Design review of the part built by this model. Coordinates are the model's own, in mm. A direction names the side the tool comes from. Give positions to 0.01 mm unless a question says otherwise; leave off trailing zeros. Loops run counter-clockwise (first coordinate to the right, second up) from the corner with the lowest first, then second, coordinate; pieces in that order, holes last.
from build123d import *

# Parameters (mm, degrees)
F1_DEPTH = 0.508
F3_DEPTH = 2.54
F5_DEPTH = 0.254


with BuildPart() as f1:
    # F0 (on Top) → F1 (new body)
    with BuildSketch(Plane.XY):
        with BuildLine():
            Line((0.5969, 12.4386211307), (0.5969, 13.7155528236))
            ThreePointArc((0.5969, 13.7155528236), (0, 20.3739569369), (-0.5969, 13.7155528236))
            Line((-0.5969, 13.7155528236), (-0.5969, 12.4386211307))
            Line((-0.5969, 12.4386211307), (-6.4008217303, 11.9018768547))
            ThreePointArc((-6.4008217303, 11.9018768547), (-6.1880330513, 11.6046108469), (-6.1128665152, 11.2468454306))
            ThreePointArc((-6.1128665152, 11.2468454306), (-6.1585456161, 10.965543349), (-6.2908886999, 10.7131493128))
            Line((-6.2908886999, 10.7131493128), (-0.5969, 11.2397270277))
            Line((-0.5969, 11.2397270277), (-0.5969, 7.3000811972))
            Line((-0.5969, 7.3000811972), (-3.5388981923, 0))
            Line((-3.5388981923, 0), (-2.2769883957, 0))
            Line((-2.2769883957, 0), (0, 5.6499695401))
            Line((0, 5.6499695401), (2.2769883957, 0))
            Line((2.2769883957, 0), (3.5388981923, 0))
            Line((3.5388981923, 0), (0.5969, 7.3000811972))
            Line((0.5969, 7.3000811972), (0.5969, 11.2397270277))
            Line((0.5969, 11.2397270277), (6.2908886999, 10.7131493128))
            ThreePointArc((6.2908886999, 10.7131493128), (6.1166438776, 11.3287104532), (6.4008217303, 11.9018768547))
            Line((6.4008217303, 11.9018768547), (0.5969, 12.4386211307))
        make_face()
        with BuildLine():
            ThreePointArc((7.8908665152, 11.2468454306), (7.3596319315, 12.0606788944), (6.4008217303, 11.9018768547))
            Line((6.4008217303, 11.9018768547), (7.0568330304, 11.8412092015))
            Line((7.0568330304, 11.8412092015), (6.9469, 10.6524816596))
            Line((6.9469, 10.6524816596), (6.2908886999, 10.7131493128))
            ThreePointArc((6.2908886999, 10.7131493128), (7.2831685968, 10.4035245315), (7.8908665152, 11.2468454306))
        make_face()
        with BuildLine():
            Line((7.0568330304, 11.8412092015), (6.4008217303, 11.9018768547))
            ThreePointArc((6.4008217303, 11.9018768547), (6.1166438776, 11.3287104532), (6.2908886999, 10.7131493128))
            Line((6.2908886999, 10.7131493128), (6.9469, 10.6524816596))
            Line((6.9469, 10.6524816596), (7.0568330304, 11.8412092015))
        make_face()
        with BuildLine():
            ThreePointArc((-6.1128665152, 11.2468454306), (-6.1880330513, 11.6046108469), (-6.4008217303, 11.9018768547))
            Line((-6.4008217303, 11.9018768547), (-7.0568330304, 11.8412092015))
            Line((-7.0568330304, 11.8412092015), (-6.9469, 10.6524816596))
            Line((-6.9469, 10.6524816596), (-6.2908886999, 10.7131493128))
            ThreePointArc((-6.2908886999, 10.7131493128), (-6.1585456161, 10.965543349), (-6.1128665152, 11.2468454306))
        make_face()
        with BuildLine():
            Line((-7.0568330304, 11.8412092015), (-6.4008217303, 11.9018768547))
            ThreePointArc((-6.4008217303, 11.9018768547), (-7.8870891528, 11.164980408), (-6.2908886999, 10.7131493128))
            Line((-6.2908886999, 10.7131493128), (-6.9469, 10.6524816596))
            Line((-6.9469, 10.6524816596), (-7.0568330304, 11.8412092015))
        make_face()
    extrude(amount=F1_DEPTH)

    # F2 (on face) → F3 (join)
    with BuildSketch(Plane.XY.offset(0.508)):
        with BuildLine():
            Line((-3.5388981923, 0), (-2.2769883957, 0))
            ThreePointArc((-2.2769883957, 0), (-2.907943294, 0.6309548983), (-3.5388981923, 0))
        make_face()
        with BuildLine():
            ThreePointArc((3.5388981923, 0), (2.907943294, 0.6309548983), (2.2769883957, 0))
            Line((2.2769883957, 0), (3.5388981923, 0))
        make_face()
    extrude(amount=F3_DEPTH)

    # F4 (on face) → F5 (join)
    with BuildSketch(Plane.XY.offset(0.508)):
        with BuildLine():
            add(Edge.make_bspline(
                [(-0.6474794169, 17.9513804615), (-0.6474794169, 18.8312622717), (-1.7904794169, 18.3913213666), (-2.9334794169, 17.9513804615), (-1.7904794169, 17.5114395563), (-0.6474794169, 17.0714986512), (-0.6474794169, 17.9513804615)],
                knots=[0, 0, 0, 2.0943951024, 2.0943951024, 4.1887902048, 4.1887902048, 6.2831853072, 6.2831853072, 6.2831853072], degree=2, weights=[1, 0.5, 1, 0.5, 1, 0.5, 1]))
        make_face()
        with BuildLine():
            add(Edge.make_bspline(
                [(0.6474794169, 17.9513804615), (0.6474794169, 17.0714986512), (1.7904794169, 17.5114395563), (2.9334794169, 17.9513804615), (1.7904794169, 18.3913213666), (0.6474794169, 18.8312622717), (0.6474794169, 17.9513804615)],
                knots=[0, 0, 0, 2.0943951024, 2.0943951024, 4.1887902048, 4.1887902048, 6.2831853072, 6.2831853072, 6.2831853072], degree=2, weights=[1, 0.5, 1, 0.5, 1, 0.5, 1]))
        make_face()
    extrude(amount=F5_DEPTH)


solid = f1.part
Q1. Wall thickness on line 1 (Z direction, x = 0, y = 10.75); line 2 (Y direction, x = 2.5, z = 1.25); line 3 (Y direction, x = -4, z = 0.2) (3 decimals): over which ranges is each line inside the solid? List them lowest first.
Results:
line 1: z = 0 to 0.51
line 2: y = 0 to 0.48
line 3: y = 10.925 to 12.124
Q2. Take a section at A-A (z = 1.65). Give the boundary of the cut face in (x, y).
Results:
outline: (-3.54, 0) - (-2.28, 0) arc R0.63 ccw to start; (2.28, 0) - (3.54, 0) arc R0.63 ccw to start
Q3. Take a section at B-B (y = 5). Give the boundary of the cut face in (x, z).
Results:
outline: (-1.52, 0) - (-0.26, 0) - (-0.26, 0.51) - (-1.52, 0.51) - close; (0.26, 0) - (1.52, 0) - (1.52, 0.51) - (0.26, 0.51) - close
Q4. Draft analysis for pull direction Y (two halves, no side actions). For faces 1 (the face through (0.14, 20.37, 0.25)), 2 (the face through (2.09, 3.6, 0.25)), 3 (the face through (-3, 0, 2)), 4 (the face through (2.92, 0.63, 1.76)), state which applies: pulls with the +Y half, pulls with the -Y half, needs draft (parallel to the pull), parting line crosses it, or undercut.
Results:
face 1: undercut
face 2: undercut
face 3: pulls with the -Y half
face 4: pulls with the +Y half
Q5. Take a section at C-C (y = 9.5). Give the boundary of the cut face in (x, z).
Results:
outline: (-0.6, 0) - (0.6, 0) - (0.6, 0.51) - (-0.6, 0.51) - close
Q6. Insertion check: pin 1 (0.6 mm diameter, centred on y = 8.5, z = 0, fed in from -X); pin 2 (0.5 mm diameter, centred on x = 1.5, y = 18, fed in from +Z). Each pin has a flat end and moves straight along its axis. Give the tip position at first contact, or say it passes through.
Results:
pin 1: stops at x = -0.6
pin 2: stops at z = 0.76
Q7. Tool access review of faces 5 (the face through (-2.89, 0.63, 1.76)), 6 (the face through (1.123, 2.865, 0.25)), 7 (the face through (3, 0, 2)): name each direction out of +Z, -Z, +X, -X, +Y, -Y from which nothing blocks a thin tool from reaching the whole face with its end or side.
Results:
face 5: +Z, +Y
face 6: +Z, -Z, -Y
face 7: +Z, -Z, +X, -X, -Y
Q8. Take a section at D-D (y = 14.75). Give the boundary of the cut face in (x, z), plus the area to 3 significant figures.
Results:
outline: (-2.47, 0) - (2.47, 0) - (2.47, 0.51) - (-2.47, 0.51) - close
area: 2.51 mm2
